Solid Edge part; units mm, degrees
sketch "Sketch1" plane through (0, 0, 0) normal (1, 0, 0) x (0, 1, 0)
  line L0 (2.4, -4.8) -> (10.9, -4.8)
  line L1 (10.9, -4.8) -> (10.9, -3.8)
  arc A0 (10.9, -3.8) -> (9.25, -1.7488) centre (11.35, -1.7488) cw
  line L2 (9.25, 0) -> (9.25, -1.7488)
  line L3 (9.25, 0) -> (9.25, 1.7488)
  arc A1 (10.9, 3.8) -> (9.25, 1.7488) centre (11.35, 1.7488) ccw
  line L4 (10.9, 4.8) -> (10.9, 3.8)
  line L5 (2.4, 4.8) -> (10.9, 4.8)
  line L6 (2.4, -4.8) -> (2.4, 4.8)
revolve "RevolvedProtrusion1" add sketch "Sketch1" angle 360 about axis through (0, 0, 0) along (0, 0, 1)
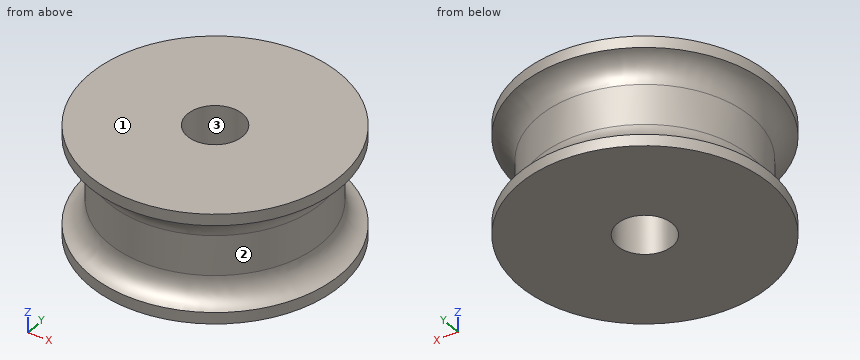
Read the model definition and answer for the solid it produces. Units are mm, in the model's axes. Face numbers are marked on the shaded views. Give positions to 0.01 mm unless a question says otherwise; leave off trailing zeros. Write each loop counter-clockwise with the first axis right and the second up, starting at its lowest first coordinate (ties: lowest second). Pieces come first, ordered by that corner, then holes. Notation, with made-up numbers: (30.5, 2.5) - (84.5, 2.5) arc R15 ccw to (84.5, 17.5) - close; hole circle Ø4 at (-33, 63). An arc over 180 degrees is marked (long way). Write item = value, one per line. Start each with the question number.
Item 1: This flat-tipped pin is pushed along its axis until it touches: P1, Ø3, axis at x = -7.5, z = 2.5, coming from the +Y side. Where does it stop, or does it pass through?
Item 2: The mould has two halves that part along Y. Classify the marked faces 1, 2 and 3: +Y half, -Y half, draft (parallel to the pull), parting line (faces both ways), or undercut.
Item 3: Find section C-C (z = 1.25). Give the vertices of the cut face in (x, y).
Item 4: Find the intervals of material crossed by probe 1 along Y at (x, z) = (0, -1.25), in increasing order. Write a range as [from, to].
Item 5: Find section A-A (x = 0). Give the vertices of the cut face in (y, z), then the cut area to 3 significant figures.
Item 6: Find section D-D (z = 3.25). Give the vertices of the cut face in (x, y), then the cut area to 3 significant figures.
Response:
q1.P1 = 8.56
q2.face_1 = draft
q2.face_2 = parting line
q2.face_3 = undercut
q3.outline = circle Ø18.5 at (0, 0); hole circle Ø4.8 at (0, 0)
q4.probe_1 = [-9.25, -2.4], [2.4, 9.25]
q5.outline = (-10.9, -4.8) - (-2.4, -4.8) - (-2.4, 4.8) - (-10.9, 4.8) - (-10.9, 3.8) arc R2.1 cw to (-9.25, 1.75) - (-9.25, -1.75) arc R2.1 cw to (-10.9, -3.8) - close; (2.4, -4.8) - (10.9, -4.8) - (10.9, -3.8) arc R2.1 cw to (9.25, -1.75) - (9.25, 1.75) arc R2.1 cw to (10.9, 3.8) - (10.9, 4.8) - (2.4, 4.8) - close
q5.area = 142 mm²
q6.outline = circle Ø19.76 at (0, 0); hole circle Ø4.8 at (0, 0)
q6.area = 289 mm²
